```python
from build123d import *

# Parameters (mm, degrees)
EXTRUDE_1_DEPTH        = 4
SM_EDGE_FLANGE_1_DEPTH = 30
FILLET_1_R             = 4
SKETCH_27_R            = 1.6
CUT_EXTRUDE_1_DEPTH    = 10
M4X0_7_1_D             = 3.3


# Sheet-metal steps are written as plain solids
with BuildPart() as part:
    # Sketch 1 → 填料-伸長1 (new body)
    with BuildSketch(Plane.XY):
        Polygon((8, 0), (8, -22), (49.5, -22), (49.5, 0), (57.5, 0), (57.5, -30), (8, -30), (0, -30), (0, 0), align=None)
    extrude(amount=EXTRUDE_1_DEPTH)

    # 邊線-凸緣1 section (across the edge) → 邊線-凸緣1 (add)
    with BuildSketch(Plane(origin=(-2, 0, 4), x_dir=(1, 0, 0), z_dir=(0, -1, 0))):
        with BuildLine():
            Line((-4, 2), (-4, 21))
            Line((-4, 21), (0, 21))
            Line((0, 21), (0, 2))
            ThreePointArc((0, 2), (0.585786438, 0.585786438), (2, 0))
            Line((2, 0), (2, -4))
            ThreePointArc((2, -4), (-2.242640687, -2.242640687), (-4, 2))
        make_face()
    extrude(amount=SM_EDGE_FLANGE_1_DEPTH)

    # 圓角1
    fillet_1_edges = [part.edges().sort_by_distance(p)[0] for p in [
        (57.5, -30, 2),
        (57.5, 0, 2),
        (49.5, 0, 2),
        (8, 0, 2),
        (-4, 0, 25),
        (-4, -30, 25),
    ]]
    fillet(fillet_1_edges, radius=FILLET_1_R - 0.0001)  # a hair under: the kernel refuses the full size

    # 草圖27 → 除料-伸長1 (cut)
    with BuildSketch(Plane(origin=(-2, 0, 0), x_dir=(0, 0, -1), z_dir=(1, 0, 0))):
        with Locations((-21, -26)):
            Circle(SKETCH_27_R)
        with Locations((-11, -26)):
            Circle(SKETCH_27_R)
        with Locations((-11, -6)):
            Circle(SKETCH_27_R)
        with Locations((-21, -6)):
            Circle(SKETCH_27_R)
    extrude(amount=-CUT_EXTRUDE_1_DEPTH, mode=Mode.SUBTRACT)

    # M4x0.7 螺紋孔1 (through all)
    with Locations(Plane(origin=(53.5, -4, 0), x_dir=(-1, 0, 0), z_dir=(0, 0, -1))):
        with Locations((0, 0), (0, -10), (49.5, 0), (49.5, -10)):
            Hole(M4X0_7_1_D / 2)


solid = part.part
```
CAD build for the part. Positions are in the model's coordinates, mm. A direction names the side the tool comes from. Coordinates: 2 decimals unless noted, no trailing zeros. Order: outer loops, then holes, each group sorted by start corner. A loop starts at its lowest first (then second) coordinate and runs counter-clockwise, first axis right, second up. Notation, with made-up numbers: M -26.5,-31.75 L -16.5,-31.75 A16 ccw -16.5,-11.75 Z; hole C 2.25,-4.75 d2. An arc over 180 degrees is marked long. Write each question's results on one line, items separated by ' | '. Start each with the question number.
Q1. Which spindle directions (+Z, -Z, +X, -X, +Y, -Y) get a long thin tool onto all of the face, cutting with end or side? Do faces 4 (the cylindrical face through (6.797, -1.141, 2.028)), 5 (the cylindrical face through (51.85, -13.93, 2.03)). Say none if no direction does.
Q2. Cut at B-B (z = 11). List the corners of the cut face in (x, y).
Q3. Cut at D-D (x = 17.5). List the corners of the cut face in (y, z), then the cut area to 3 significant figures.
Q4. Pull direction Y, two halves, no side cores. Call faces 1 (the flat face through (8, -13, 2)), 2 (the cylindrical face through (2.784, -12.885, 2.028)), 3 (the cylindrical face through (56.297, -1.141, 2.028)): +Y half, -Y half, draft (parallel to the pull), parting line (faces both ways), or undercut.
Q5. Drill centre lines: probe 1 along Y at (x, z) = (4, 0.8); probe 2 along X at (y, z) = (-15, 2); probe 3 along X at (y, z) = (-8, 15.75). Where is each one in solid material? Low to high. Write a range as from..to.
Q6. Cut at C-C (y = -8.75). List the corners of the cut face in (x, z), then the cut area to 3 significant figures.
Q7. Cut at A-A (y = -14). List the corners of the cut face in (x, z).
Q8. Flat gauge pins, fed straight in: P1, Ø6, axis at x = 15.5, z = 6, coming from the +Y side; P2, Ø5.5, axis at y = -16, z = 17.5, coming from the +X side; P3, Ø5.5, axis at x = 4, y = -4, coming from the +Z side. Where does each tip first touch, or does it go through?
Found:
1) face 4: +Z, -Z, +Y | face 5: +Z, -Z
2) outline: M -6,-30 L -2,-30 L -2,-27.6 L -6,-27.6 Z; M -6,-24.4 L -2,-24.4 L -2,-7.6 L -6,-7.6 Z; M -6,-4.4 L -2,-4.4 L -2,0 L -6,0 Z
3) outline: M -30,0 L -22,0 L -22,4 L -30,4 Z | area: 32.0 mm²
4) face 1: draft | face 2: undercut | face 3: +Y half
5) probe 1: -30..-15.65, -12.35..-5.65, -2.35..0 | probe 2: -4.47..2.69, 5.31..8, 49.5..52.19, 54.81..57.5 | probe 3: -6..-2
6) outline: M -6,6 A6 ccw 0,0 L 8,0 L 8,4 L 0,4 A2 cw -2,6 L -2,25 L -6,25 Z; M 49.5,0 L 57.5,0 L 57.5,4 L 49.5,4 Z | area: 165 mm²
7) outline: M -6,6 A6 ccw 0,0 L 2.35,0 L 2.35,4 L 0,4 A2 cw -2,6 L -2,25 L -6,25 Z; M 5.65,0 L 8,0 L 8,4 L 5.65,4 Z; M 49.5,0 L 51.85,0 L 51.85,4 L 49.5,4 Z; M 55.15,0 L 57.5,0 L 57.5,4 L 55.15,4 Z
8) P1: y = -22 | P2: x = -2 | P3: z = 4
